```python
from build123d import *

# Parameters (mm, degrees)
F0_W     = 120.015
F0_H     = 152.4
F0_R     = 3.175
F0_W_2   = 88.9
F0_H_2   = 6.35
F1_DEPTH = 12.7


with BuildPart() as f1:
    # F0 (on Front) → F1 (new body)
    with BuildSketch(Plane.XZ):
        with Locations((-60.0075, 76.2)):
            Rectangle(F0_W, F0_H)
        with Locations((-100.965, 6.35)):
            Circle(F0_R, mode=Mode.SUBTRACT)
        with Locations((-19.05, 6.35)):
            Circle(F0_R, mode=Mode.SUBTRACT)
        with Locations((-60.0075, 66.675)):
            Rectangle(F0_W_2, F0_H_2, mode=Mode.SUBTRACT)
        with Locations((-113.665, 79.375)):
            Circle(F0_R, mode=Mode.SUBTRACT)
        with Locations((-113.665, 136.525)):
            Circle(F0_R, mode=Mode.SUBTRACT)
        with Locations((-6.35, 79.375)):
            Circle(F0_R, mode=Mode.SUBTRACT)
        with Locations((-60.0075, 118.745)):
            Rectangle(F0_W_2, F0_H_2, mode=Mode.SUBTRACT)
        with Locations((-6.35, 136.525)):
            Circle(F0_R, mode=Mode.SUBTRACT)
    extrude(amount=F1_DEPTH)


solid = f1.part
```
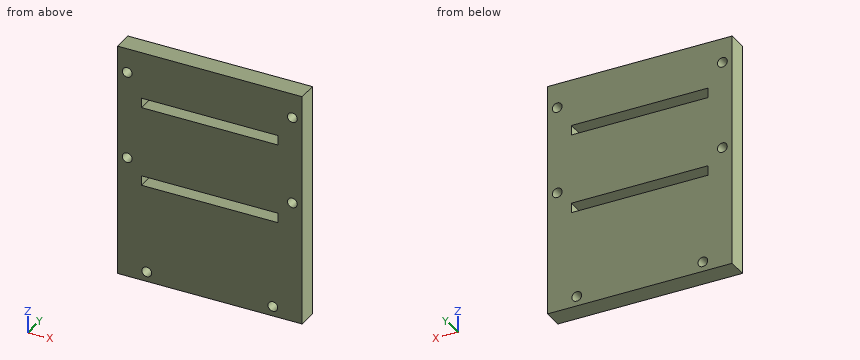
Part model, mm, in its own coordinate system. Give positions to 0.01 mm unless a question says otherwise; leave off trailing zeros. Loops run counter-clockwise (first coordinate to the right, second up) from the corner with the lowest first, then second, coordinate; pieces in that order, holes last. Notation, with made-up numbers: M -9,-38.5 L 44,-38.5 A35 ccw 44,-6.5 Z; hole C -31.75,69.25 d5. An arc over 180 degrees is marked long. Return JSON: item names as keys, results as strings.
1) Saw through at C-C, the plane x = -6.35. List the corners of the cut face in (y, z).
Calculated:
{"outline": "M -12.7,0 L 0,0 L 0,76.2 L -12.7,76.2 Z; M -12.7,82.55 L 0,82.55 L 0,133.35 L -12.7,133.35 Z; M -12.7,139.7 L 0,139.7 L 0,152.4 L -12.7,152.4 Z"}
2) Saw through at D-D, the plane y = -5.5. Count the separate pieces of the cut face and the enclosed holes in it, then the cut area to 3 significant figures.
Calculated:
{"separate pieces": "1", "enclosed holes": "8", "area": "17,000 mm2"}
3) Drill centre lines: line 1 (Z direction, x = -6.35, y = -9.5); line 2 (Z direction, x = -60.5, y = -4.25); line 3 (Z direction, x = -19.05, y = -5.75) (3 decimals). Where is each one in solid material? Low to high.
Calculated:
{"line 1": "z = 0 to 76.2, 82.55 to 133.35, 139.7 to 152.4", "line 2": "z = 0 to 63.5, 69.85 to 115.57, 121.92 to 152.4", "line 3": "z = 0 to 3.175, 9.525 to 63.5, 69.85 to 115.57, 121.92 to 152.4"}
4) Saw through at B-B, the plane z = 6.35. List the corners of the cut face in (x, y) (3 decimals), then the cut area to 3 significant figures.
Calculated:
{"outline": "M -120.015,-12.7 L -104.14,-12.7 L -104.14,0 L -120.015,0 Z; M -97.79,-12.7 L -22.225,-12.7 L -22.225,0 L -97.79,0 Z; M -15.875,-12.7 L 0,-12.7 L 0,0 L -15.875,0 Z", "area": "1,360 mm2"}
5) Saw through at A-A, the plane x = -19.05. List the corners of the cut face in (y, z) (3 decimals), then the cut area to 3 significant figures.
Calculated:
{"outline": "M -12.7,0 L 0,0 L 0,3.175 L -12.7,3.175 Z; M -12.7,9.525 L 0,9.525 L 0,63.5 L -12.7,63.5 Z; M -12.7,69.85 L 0,69.85 L 0,115.57 L -12.7,115.57 Z; M -12.7,121.92 L 0,121.92 L 0,152.4 L -12.7,152.4 Z", "area": "1,690 mm2"}
